Can you work these out from the model? Positions are in its coordinate system, mm. Face numbers are marked on the shaded views. A direction names the side the tool comes from. Round coordinates to 2 decimals unless told otherwise and drop trailing zeros. Loops run counter-clockwise (first coordinate to the right, second up) from the corner with the lowest first, then second, coordinate; pieces in that order, holes last. Notation, with made-up numbers: (-39, -9.5) -> (13, -9.5) arc R25 ccw to (13, 15.5) -> close; hole circle Ø5 at (84.25, 29.5). An arc over 180 degrees is marked (long way). Write each question's results on one line, items separated by ' | '.
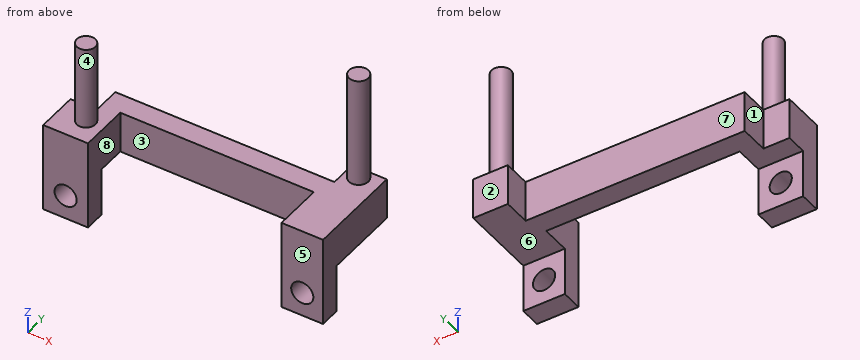
from build123d import *

# Parameters (mm, degrees)
SKETCH1_W            = 4
SKETCH1_H            = 14
BOSS_EXTRUDE1_DEPTH  = 3
SKETCH2_R            = 1.4
BOSS_EXTRUDE2_DEPTH  = 16
SKETCH3_W            = 4
SKETCH3_H            = 1
BOSS_EXTRUDE4_DEPTH  = 6
SKETCH7_W            = 3
SKETCH7_H            = 2
BOSS_EXTRUDE5_DEPTH  = 30.95
SKETCH8_W            = 3
SKETCH8_H            = 2
BOSS_EXTRUDE6_DEPTH  = 1
SKETCH9_W            = 1
SKETCH9_H            = 2
BOSS_EXTRUDE7_DEPTH  = 3
SKETCH10_W           = 1
SKETCH10_H           = 2
BOSS_EXTRUDE8_DEPTH  = 5.92
SKETCH11_W           = 1
SKETCH11_H           = 2
BOSS_EXTRUDE9_DEPTH  = 4
SKETCH12_W           = 1
SKETCH12_H           = 3
BOSS_EXTRUDE14_DEPTH = 0.93
SKETCH13_W           = 3
SKETCH13_H           = 3
BOSS_EXTRUDE15_DEPTH = 7.1
SKETCH14_W           = 3.33402541
SKETCH14_H           = 13.860919233
CUT_EXTRUDE3_DEPTH   = 10
SKETCH15_W           = 6.20666024
SKETCH15_H           = 3.660501205
CUT_EXTRUDE4_DEPTH   = 10
SKETCH16_W           = 3
SKETCH16_H           = 9.1
BOSS_EXTRUDE16_DEPTH = 0.12
SKETCH18_W           = 3
SKETCH18_H           = 9.1
BOSS_EXTRUDE18_DEPTH = 0.41
SKETCH19_W           = 3
SKETCH19_H           = 9.1
BOSS_EXTRUDE19_DEPTH = 0.89
SKETCH20_W           = 3
SKETCH20_H           = 6
BOSS_EXTRUDE20_DEPTH = 3.77
SKETCH21_R           = 1.35
BOSS_EXTRUDE23_DEPTH = 12
BOSS_EXTRUDE24_DEPTH = 3
SKETCH24_W           = 4
SKETCH24_H           = 1
BOSS_EXTRUDE25_DEPTH = 4
SKETCH25_W           = 4
SKETCH25_H           = 7
BOSS_EXTRUDE26_DEPTH = 2
SKETCH26_W           = 6.458993184
SKETCH26_H           = 3
BOSS_EXTRUDE27_DEPTH = 7
SKETCH27_R           = 1.6
CUT_EXTRUDE5_DEPTH   = 7
SKETCH28_R           = 1.6
CUT_EXTRUDE6_DEPTH   = 7
SKETCH30_W           = 7
SKETCH30_H           = 3
BOSS_EXTRUDE29_DEPTH = 1
SKETCH31_W           = 7
SKETCH31_H           = 3
BOSS_EXTRUDE30_DEPTH = 1
SKETCH32_W           = 6
SKETCH32_H           = 7.1
BOSS_EXTRUDE31_DEPTH = 1
SKETCH33_W           = 31.638993184
SKETCH33_H           = 6
BOSS_EXTRUDE32_DEPTH = 1
SKETCH34_W           = 6
SKETCH34_H           = 14
BOSS_EXTRUDE33_DEPTH = 1


with BuildPart() as part:
    # Sketch1 → Boss-Extrude1 (new body)
    with BuildSketch(Plane.XY):
        with Locations((-1.434146341, -3.597560976)):
            Rectangle(SKETCH1_W, SKETCH1_H)
    extrude(amount=BOSS_EXTRUDE1_DEPTH)

    # Sketch2 → Boss-Extrude2 (add)
    with BuildSketch(Plane(origin=(0, 0, 0), x_dir=(-1, 0, 0), z_dir=(0, 0, -1))):
        with Locations(Location((1.434146341, 1.802439024, 0), (0, 0, 180))):
            Circle(SKETCH2_R)
    extrude(amount=BOSS_EXTRUDE2_DEPTH)

    # Sketch3 → Boss-Extrude4 (add)
    with BuildSketch(Plane.XY.offset(3)):
        with Locations((-1.434146341, -10.097560976)):
            Rectangle(SKETCH3_W, SKETCH3_H)
    extrude(amount=BOSS_EXTRUDE4_DEPTH)

    # Sketch7 → Boss-Extrude5 (add)
    with BuildSketch(Plane.ZY.offset(3.434146341)):
        with Locations((1.5, -2.497560976)):
            Rectangle(SKETCH7_W, SKETCH7_H)
    extrude(amount=BOSS_EXTRUDE5_DEPTH)

    # Sketch8 → Boss-Extrude6 (add)
    with BuildSketch(Plane.ZY.offset(34.384146341)):
        with Locations((1.5, -2.497560976)):
            Rectangle(SKETCH8_W, SKETCH8_H)
    extrude(amount=BOSS_EXTRUDE6_DEPTH)

    # Sketch9 → Boss-Extrude7 (add)
    with BuildSketch(Plane(origin=(0, 0, 0), x_dir=(-1, 0, 0), z_dir=(0, 0, -1))):
        with Locations((34.884146341, -2.497560976)):
            Rectangle(SKETCH9_W, SKETCH9_H)
    extrude(amount=BOSS_EXTRUDE7_DEPTH)

    # Sketch10 → Boss-Extrude8 (add)
    with BuildSketch(Plane(origin=(0, 0, -3), x_dir=(-1, 0, 0), z_dir=(0, 0, -1))):
        with Locations((34.884146341, -2.497560976)):
            Rectangle(SKETCH10_W, SKETCH10_H)
    extrude(amount=BOSS_EXTRUDE8_DEPTH)

    # Sketch11 → Boss-Extrude9 (add)
    with BuildSketch(Plane(origin=(0, 0, -8.92), x_dir=(-1, 0, 0), z_dir=(0, 0, -1))):
        with Locations((34.884146341, -2.497560976)):
            Rectangle(SKETCH11_W, SKETCH11_H)
    extrude(amount=BOSS_EXTRUDE9_DEPTH)

    # Sketch12 → Boss-Extrude14 (add)
    with BuildSketch(Plane.XZ.offset(3.497560976)):
        with Locations((-34.884146341, -9.28)):
            Rectangle(SKETCH12_W, SKETCH12_H)
    extrude(amount=BOSS_EXTRUDE14_DEPTH)

    # Sketch13 → Boss-Extrude15 (add)
    with BuildSketch(Plane.XZ.offset(3.497560976)):
        with Locations((-33.884146341, 1.5)):
            Rectangle(SKETCH13_W, SKETCH13_H)
    extrude(amount=BOSS_EXTRUDE15_DEPTH)

    # Sketch14 → Cut-Extrude3 (cut)
    with BuildSketch(Plane.XY.offset(3)):
        with Locations((-35.32015223, -3.66710136)):
            Rectangle(SKETCH14_W, SKETCH14_H)
    extrude(amount=-CUT_EXTRUDE3_DEPTH, mode=Mode.SUBTRACT)


with BuildPart() as cut_extrude3_piece_1:
    # of the separate pieces the step leaves, piece 1, a body of its own (cut_extrude3_pieces)
    add(part.part.solids().sort_by_distance((-3.434146341, 3.402439024, 0))[0])

    # Sketch16 → Boss-Extrude16 (add)
    with BuildSketch(Plane.ZY.offset(33.653139525)):
        with Locations((1.5, -6.047560976)):
            Rectangle(SKETCH16_W, SKETCH16_H)
    extrude(amount=BOSS_EXTRUDE16_DEPTH)

    # Sketch18 → Boss-Extrude18 (add)
    with BuildSketch(Plane.ZY.offset(33.773139525)):
        with Locations((1.5, -6.047560976)):
            Rectangle(SKETCH18_W, SKETCH18_H)
    extrude(amount=BOSS_EXTRUDE18_DEPTH)

    # Sketch19 → Boss-Extrude19 (add)
    with BuildSketch(Plane.ZY.offset(34.183139525)):
        with Locations((1.5, -6.047560976)):
            Rectangle(SKETCH19_W, SKETCH19_H)
    extrude(amount=BOSS_EXTRUDE19_DEPTH)

    # Sketch20 → Boss-Extrude20 (add)
    with BuildSketch(Plane.ZY.offset(35.073139525)):
        with Locations((1.5, -7.597560976)):
            Rectangle(SKETCH20_W, SKETCH20_H)
    extrude(amount=BOSS_EXTRUDE20_DEPTH)

    # Sketch21 → Boss-Extrude23 (add)
    with BuildSketch(Plane(origin=(0, 0, 0), x_dir=(-1, 0, 0), z_dir=(0, 0, -1))):
        with Locations(Location((34.984146341, -7.047560976, 0), (0, 0, 180))):
            Circle(SKETCH21_R)
    extrude(amount=BOSS_EXTRUDE23_DEPTH)

    # Sketch23 → Boss-Extrude24 (add)
    with BuildSketch(Plane.XY.offset(3)):
        Polygon((-38.843139525, -10.597560976), (-38.843139525, -4.597560976), (-35.073139525, -4.597560976), (-35.073139525, -1.497560976), (-3.434146341, -1.497560976), (-3.434146341, 3.402439024), (0.565853659, 3.402439024), (0.565853659, -9.597560976), (-3.434146341, -9.597560976), (-3.434146341, -3.497560976), (-32.384146341, -3.497560976), (-32.384146341, -10.597560976), align=None)
    extrude(amount=BOSS_EXTRUDE24_DEPTH)

    # Sketch24 → Boss-Extrude25 (add)
    with BuildSketch(Plane.XY.offset(9)):
        with Locations((-1.434146341, -10.097560976)):
            Rectangle(SKETCH24_W, SKETCH24_H)
    extrude(amount=BOSS_EXTRUDE25_DEPTH)

    # Sketch25 → Boss-Extrude26 (add)
    with BuildSketch(Plane(origin=(0, -9.597560976, 0), x_dir=(1, 0, 0), z_dir=(0, 1, 0))):
        with Locations((-1.434146341, -9.5)):
            Rectangle(SKETCH25_W, SKETCH25_H)
    extrude(amount=BOSS_EXTRUDE26_DEPTH)

    # Sketch26 → Boss-Extrude27 (add)
    with BuildSketch(Plane.XY.offset(6)):
        with Locations((-35.613642933, -9.097560976)):
            Rectangle(SKETCH26_W, SKETCH26_H)
    extrude(amount=BOSS_EXTRUDE27_DEPTH)

    # Sketch27 → Cut-Extrude5 (cut)
    with BuildSketch(Plane(origin=(0, -7.597560976, 0), x_dir=(1, 0, 0), z_dir=(0, 1, 0))):
        with Locations(Location((-35.613642933, -9.5, 0), (0, 0, 270))):
            Circle(SKETCH27_R)
    extrude(amount=-CUT_EXTRUDE5_DEPTH, mode=Mode.SUBTRACT)

    # Sketch28 → Cut-Extrude6 (cut)
    with BuildSketch(Plane(origin=(0, -7.597560976, 0), x_dir=(1, 0, 0), z_dir=(0, 1, 0))):
        with Locations(Location((-1.434146341, -9.5, 0), (0, 0, 270))):
            Circle(SKETCH28_R)
    extrude(amount=-CUT_EXTRUDE6_DEPTH, mode=Mode.SUBTRACT)

    # Sketch30 → Boss-Extrude29 (add)
    with BuildSketch(Plane(origin=(0.565853659, 0, 0), x_dir=(0, 0, -1), z_dir=(1, 0, 0))):
        with Locations((-9.5, -9.097560976)):
            Rectangle(SKETCH30_W, SKETCH30_H)
    extrude(amount=BOSS_EXTRUDE29_DEPTH)

    # Sketch31 → Boss-Extrude30 (add)
    with BuildSketch(Plane.ZY.offset(3.434146341)):
        with Locations((9.5, -9.097560976)):
            Rectangle(SKETCH31_W, SKETCH31_H)
    extrude(amount=BOSS_EXTRUDE30_DEPTH)

    # Sketch32 → Boss-Extrude31 (add)
    with BuildSketch(Plane.ZY.offset(3.434146341)):
        with Locations((3, -7.047560976)):
            Rectangle(SKETCH32_W, SKETCH32_H)
    extrude(amount=BOSS_EXTRUDE31_DEPTH)

    # Sketch33 → Boss-Extrude32 (add)
    with BuildSketch(Plane(origin=(0, -1.497560976, 0), x_dir=(1, 0, 0), z_dir=(0, 1, 0))):
        with Locations((-19.253642933, -3)):
            Rectangle(SKETCH33_W, SKETCH33_H)
    extrude(amount=BOSS_EXTRUDE32_DEPTH)

    # Sketch34 → Boss-Extrude33 (add)
    with BuildSketch(Plane(origin=(0.565853659, 0, 0), x_dir=(0, 0, -1), z_dir=(1, 0, 0))):
        with Locations((-3, -3.597560976)):
            Rectangle(SKETCH34_W, SKETCH34_H)
    extrude(amount=BOSS_EXTRUDE33_DEPTH)


with BuildPart() as cut_extrude3_piece_2:
    # of the separate pieces the step leaves, piece 2, a body of its own (cut_extrude3_pieces)
    add(part.part.solids().sort_by_distance((-34.384146341, -1.497560976, -7))[0])

    # Sketch15 → Cut-Extrude4 (cut)
    with BuildSketch(Plane.ZY.offset(35.384146341)):
        with Locations((-9.81666988, -3.327811578)):
            Rectangle(SKETCH15_W, SKETCH15_H)
    extrude(amount=-CUT_EXTRUDE4_DEPTH, mode=Mode.SUBTRACT)


with BuildPart() as body_2:
    # Mirror1: mirrored copy
    add(cut_extrude3_piece_1.part.mirror(Plane.XY.offset(-86.517216343)))


solid = body_2.part
1. If we section it at C-C (x = -1): List the corners of the cut face in (y, z) for me.
Final values:
outline: (-10.6, -186.03) -> (-7.6, -186.03) -> (-7.6, -184.07) -> (-10.6, -184.07) -> close; (-10.6, -180.99) -> (-7.6, -180.99) -> (-7.6, -179.03) -> (3.4, -179.03) -> (3.4, -173.03) -> (3.13, -173.03) -> (3.13, -157.03) -> (0.47, -157.03) -> (0.47, -173.03) -> (-10.6, -173.03) -> close
2. We'd pull the mould along X, two halves only. Please class the marked faces 1, 2 and 3: pulls with the +X half, pulls with the -X half, needs draft (parallel to the pull), parting line crosses it, or undercut.
Final values:
face 1: pulls with the -X half | face 2: needs draft | face 3: undercut
3. Will these pins go through, and if not, where does the flat tip stop? pin 1 (1.8 mm diameter, centred on x = -18, z = -177.5, fed in from -Y); pin 2 (4 mm diameter, centred on x = -36.5, z = -177, fed in from +Y); pin 3 (6 mm diameter, centred on x = -13.5, y = 1, fed in from -Z).
Final values:
pin 1: y = -3.5 | pin 2: y = -0.5 | pin 3: z = -179.03
4. Please list where these lines run through material, in increasing order: line 1 (Y direction, x = -22, z = -178); line 2 (Z direction, x = -15, y = -3); line 3 (X direction, y = -4, z = -174.25). Write a range as from..to.
Final values:
line 1: -3.5..-0.5 | line 2: -179.03..-173.03 | line 3: -35.07..-32.38, -4.43..1.57
5. If we section it at D-D (y = 2.25): List the corners of the cut face in (x, z) for me, then the cut area to 3 significant figures.
Final values:
outline: (-3.43, -179.03) -> (1.57, -179.03) -> (1.57, -173.03) -> (-0.11, -173.03) -> (-0.11, -157.03) -> (-2.76, -157.03) -> (-2.76, -173.03) -> (-3.43, -173.03) -> close | area: 72.4 mm2
6. If we section it at A-A (y = -9.25): List the corners of the cut face in (x, z) for me, then the cut area to 3 significant figures.
Final values:
outline: (-38.84, -186.03) -> (-32.38, -186.03) -> (-32.38, -173.03) -> (-38.84, -173.03) -> close; (-4.43, -186.03) -> (1.57, -186.03) -> (1.57, -173.03) -> (-4.43, -173.03) -> close; hole circle Ø3.2 at (-35.61, -182.53); hole circle Ø3.2 at (-1.43, -182.53) | area: 146 mm2
7. If we section it at B-B (z = -179.75): List the corners of the cut face in (x, y) for me, then the cut area to 3 significant figures.
Final values:
outline: (-38.84, -10.6) -> (-32.38, -10.6) -> (-32.38, -7.6) -> (-38.84, -7.6) -> close; (-4.43, -10.6) -> (1.57, -10.6) -> (1.57, -7.6) -> (-4.43, -7.6) -> close | area: 37.4 mm2
8. On a 3-axis mill with a long thin cutter (end or side, diameter ignored), from which of +Z, -Z, +X, -X, +Y, -Y can I reach the whole of each face in a straight line? I mean the marked faces 4, 5, 6, 7 and 8. Say none if no direction works.
Final values:
face 4: +Z | face 5: +Z, -Z, +X, -X, -Y | face 6: -Z, +X, -X, +Y | face 7: +Z, -Z, -X, +Y | face 8: +Z, -Z, -Y
